Read the model definition and answer for the solid it produces. Units are mm, in the model's axes. Coordinates: 2 decimals unless noted, no trailing zeros. Loops run counter-clockwise (first coordinate to the right, second up) from the corner with the lowest first, then second, coordinate; pieces in that order, holes last.
Solid Edge part; units mm, degrees
sketch "Sketch1" plane through (0, 0, 0) normal (0, 0, 1) x (1, 0, 0)
  line L0 (0, 10.6667) -> (0, 6)
  line L1 (0, 6) -> (27.4, 6)
  line L2 (27.4, 6) -> (27.4, 10.6667)
  line L3 (27.4, 10.6667) -> (14.7489, 10.6667)
  arc A0 (14.7489, 10.6667) -> (8.2511, 10.6667) centre (11.5, 13) cw
  line L4 (8.2511, 10.6667) -> (0, 10.6667)
revolve "RevolvedProtrusion1" add sketch "Sketch1" angle 360 about axis through (27.4, 0, 0) along (-1, 0, 0)
sketch "Sketch2" plane through (0, 0, 0) normal (0, -1, 0) x (1, 0, 0)
  circle A0 centre (23.4, 0) radius 3
extrude "Cutout1" cut sketch "Sketch2" against normal blind 40
properties part number "UCP201 GB/T7810-1995_PART2"
Q1. Straight lines are drawn through the part: probe 1 along Z at (x, y) = (19, 0); probe 2 along X at (y, z) = (8.95, 0); probe 3 along Y at (x, z) = (4, 1). For each, find the intervals that lie inside material, in ascending order.
Findings below:
probe 1: z = -10.67 to -6, 6 to 10.67
probe 2: x = 0 to 20.4, 26.4 to 27.4
probe 3: y = -10.62 to -5.92, 5.92 to 10.62
Q2. A cutting plane is placed at B-B (z = 0). Give the vertices of the cut face in (x, y).
Findings below:
outline: (0, -10.67) - (8.25, -10.67) arc R4 cw to (14.75, -10.67) - (27.4, -10.67) - (27.4, -6) - (0, -6) - close; (0, 6) - (20.4, 6) - (20.4, 10.67) - (14.75, 10.67) arc R4 cw to (8.25, 10.67) - (0, 10.67) - close; (26.4, 6) - (27.4, 6) - (27.4, 10.67) - (26.4, 10.67) - close
Q3. A cutting plane is placed at D-D (x = 23.4). Give the vertices of the cut face in (y, z), then the cut area to 3 significant figures.
Findings below:
outline: (5.2, -3) arc R6 cw (long way) to (5.2, 3) - (10.24, 3) arc R10.67 ccw (long way) to (10.24, -3) - close
area: 216 mm2
Q4. Flat-ended cylindrical pins translate along their axes: pin 1 Ø10 at (x, z) = (9.5, -7.5) entering from +Y; pin 2 Ø5 at (x, z) = (19, -7.5) entering from +Y; pin 3 Ø5 at (x, y) = (13, 3) entering from +Z. Find the tip coordinate at first contact, or state that the pin passes through.
Findings below:
pin 1: stops at y = 10.33
pin 2: stops at y = 9.42
pin 3: stops at z = 10.6
Q5. A cutting plane is placed at C-C (x = 18.5). Give the vertices of the cut face in (y, z), then the cut area to 3 significant figures.
Findings below:
outline: circle Ø21.33 at (0, 0); hole circle Ø12 at (0, 0)
area: 244 mm2
Q6. A cutting plane is placed at A-A (y = 0). Give the vertices of the cut face in (x, z).
Findings below:
outline: (0, -10.67) - (8.25, -10.67) arc R4 cw to (14.75, -10.67) - (27.4, -10.67) - (27.4, -6) - (0, -6) - close; (0, 6) - (27.4, 6) - (27.4, 10.67) - (14.75, 10.67) arc R4 cw to (8.25, 10.67) - (0, 10.67) - close
Q7. Determine the mould class of faces 1 (the face through (0, 5, 5)), 2 (the face through (27.4, 5, 5)), 3 (the face through (26.17, 7.89, -1.15)) for opening direction X: +X half, -X half, draft (parallel to the pull), parting line (faces both ways), or undercut.
Findings below:
face 1: -X half
face 2: +X half
face 3: undercut
